Here's how the part is built. I have some questions about the finished solid (model axes, mm). A direction names the side the tool comes from. Round coordinates to 2 decimals unless told otherwise and drop trailing zeros. Order: outer loops, then holes, each group sorted by start corner. A loop starts at its lowest first (then second) coordinate and runs counter-clockwise, first axis right, second up. Notation, with made-up numbers: (-18.5, 72) -> (15.5, 72) arc R31 cw to (15.5, 103) -> close; hole circle Ø9 at (37, -3). An arc over 180 degrees is marked (long way). Use a Markdown table: item, result. Add a question column.
(1) I want a section at B-B, the plane z = 91. Please give me the cut outline in (x, y).
(2) If I drill on probe 1 along Z at (x, y) = (-15, -3.7); probe 2 along Z at (x, y) = (15, -5); probe 3 along Z at (x, y) = (12, -0.25), over which ranges is the centre line in solid material (lowest first)?
(3) On a 3-axis mill with a long thin cutter (end or side, diameter ignored), from which of +Z, -Z, +X, -X, +Y, -Y can I reach the whole of each face in a straight line? I mean faces 4 (the face through (21, -12, 48)), 5 (the face through (9.5, -5, 6)), 6 (the face through (-4, -6, 75.5)), 7 (the face through (0, -6.2, 47.5)), 8 (the face through (-13.9, -3, 33.9)). Say none if no direction works.
(4) I'm going to push flat-ended pins straight in: P1, Ø2, axis at y = -8.5, z = 70.5, coming from the -X side; P2, Ø6, axis at x = 12.5, z = 20, coming from the -Y side; P3, Ø3.5, axis at x = -4, y = -9, coming from the +Z side. Where does each tip first touch, or does it pass through?
(5) I want a section at C-C, the plane x = 0. Please give me the cut outline in (y, z), then the cut area to 3 significant figures.
(6) Thinking about a two-plate mould opening in X: for faces 1 (the face through (-21.843, -2, 48)), 2 (the face through (-13.6, -1.48, 62.06)), 3 (the face through (-17, -4, 48)), which applies, pulls with the +X half, pulls with the -X half, needs draft (parallel to the pull), parting line crosses it, or undercut?
(7) I want a section at D-D, the plane z = 62. Please give me the cut outline in (x, y).
(8) I want a section at A-A, the plane x = 15. Please give me the cut outline in (y, z).
from build123d import *

# Parameters (mm, degrees)
SKETCH012_R  = 4
PAD008_DEPTH = 12
SKETCH001_R  = 1.4
SKETCH001_W  = 29.46
SKETCH001_H  = 21.5
PAD005_DEPTH = 13
PAD006_DEPTH = 24
SKETCH010_R  = 2.5
PAD007_DEPTH = 4
SKETCH011_R  = 2.5
PAD004_DEPTH = 1
PAD001_DEPTH = 1
PAD002_DEPTH = 2
PAD003_DEPTH = 1
PAD_DEPTH    = 97


with BuildPart() as pad008:
    # Sketch012 → Pad008 (new body)
    with BuildSketch(Plane.XZ):
        with Locations((30, 65)):
            Circle(SKETCH012_R)
    extrude(amount=PAD008_DEPTH)


with BuildPart() as pad005:
    # Sketch001 → Pad005 (new body)
    with BuildSketch(Plane(origin=(0, 0, 0), x_dir=(-1, 0, 0), z_dir=(0, 1, 0))):
        with Locations((15, 62)):
            Circle(SKETCH001_R)
        with Locations((15, 35)):
            Circle(SKETCH001_R)
        with Locations((-15, 62)):
            Circle(SKETCH001_R)
        with Locations((-15, 35)):
            Circle(SKETCH001_R)
        with Locations((7.27, 10.75)):
            Rectangle(SKETCH001_W, SKETCH001_H)
        with Locations((7.27, 86.25)):
            Rectangle(SKETCH001_W, SKETCH001_H)
    extrude(amount=-PAD005_DEPTH)


with BuildPart() as pad006:
    # Sketch008 → Pad006 (new body)
    with BuildSketch(Plane.YZ.offset(33.5)):
        with BuildLine():
            ThreePointArc((-1, 7.5), (-8.915757, 6), (-1, 4.5))
            Line((0, 4.5), (-1, 4.5))
            Line((0, 7.5), (0, 4.5))
            Line((-1, 7.5), (0, 7.5))
        make_face()
        with BuildLine():
            ThreePointArc((-1, 92.5), (-8.915757, 91), (-1, 89.5))
            Line((0, 89.5), (-1, 89.5))
            Line((0, 92.5), (0, 89.5))
            Line((-1, 92.5), (0, 92.5))
        make_face()
    extrude(amount=-PAD006_DEPTH)


with BuildPart() as pad007:
    # Sketch010 → Pad007 (new body)
    with BuildSketch(Plane.XZ.offset(12)):
        with Locations((15, 62)):
            Circle(SKETCH010_R)
        with Locations((15, 35)):
            Circle(SKETCH010_R)
    extrude(amount=-PAD007_DEPTH)


with BuildPart() as cutblock:
    # Sketch011 → Pad004 (new body)
    with BuildSketch(Plane.XZ.offset(4)):
        with Locations((-15, 62)):
            Circle(SKETCH011_R)
        with Locations((-15, 35)):
            Circle(SKETCH011_R)
    extrude(amount=-PAD004_DEPTH)

    # Fusion001: union Pad005, Pad006, Pad007
    add(pad005.part)
    add(pad006.part)
    add(pad007.part)


with BuildPart() as pad001:
    # Sketch005 → Pad001 (new body)
    with BuildSketch(Plane(origin=(0, 0, 21.5), x_dir=(-1, 0, 0), z_dir=(0, 0, 1))):
        with BuildLine():
            ThreePointArc((7.46, 0), (0, 7.46), (-7.46, 0))
            Line((-7.46, 0), (-6, 0))
            ThreePointArc((6, 0), (0, 6), (-6, 0))
            Line((7.46, 0), (6, 0))
        make_face()
    extrude(amount=PAD001_DEPTH)


with BuildPart() as pad002:
    # Sketch006 → Pad002 (new body)
    with BuildSketch(Plane(origin=(0, 0, 47.5), x_dir=(-1, 0, 0), z_dir=(0, 0, 1))):
        with BuildLine():
            ThreePointArc((7.46, 0), (0, 7.46), (-7.46, 0))
            Line((-7.46, 0), (-6, 0))
            ThreePointArc((6, 0), (0, 6), (-6, 0))
            Line((7.46, 0), (6, 0))
        make_face()
    extrude(amount=PAD002_DEPTH)


with BuildPart() as pad003:
    # Sketch007 → Pad003 (new body)
    with BuildSketch(Plane(origin=(0, 0, 74.5), x_dir=(-1, 0, 0), z_dir=(0, 0, 1))):
        with BuildLine():
            ThreePointArc((7.46, 0), (0, 7.46), (-7.46, 0))
            Line((-7.46, 0), (-6, 0))
            ThreePointArc((6, 0), (0, 6), (-6, 0))
            Line((7.46, 0), (6, 0))
        make_face()
    extrude(amount=PAD003_DEPTH)


with BuildPart() as cut001:
    # Sketch → Pad (new body)
    with BuildSketch(Plane.XY):
        with BuildLine():
            ThreePointArc((-7.46, 0), (0, -7.46), (7.46, 0))
            Line((7.46, 0), (40, 0))
            Line((40, -12), (40, 0))
            Line((3.5, -12), (40, -12))
            ThreePointArc((-11.842719, -4), (-5.779294, -11.083761), (3.5, -12))
            Line((-21.842719, -4), (-11.842719, -4))
            Line((-21.842719, 0), (-21.842719, -4))
            Line((-7.46, 0), (-21.842719, 0))
        make_face()
    extrude(amount=PAD_DEPTH)

    # Fusion: union Pad001, Pad002, Pad003
    add(pad001.part)
    add(pad002.part)
    add(pad003.part)

    # Cut: cut CutBlock
    add(cutblock.part, mode=Mode.SUBTRACT)

    # Cut001: cut Pad008
    add(pad008.part, mode=Mode.SUBTRACT)


solid = cut001.part
Taken from the geometry:
| question | item | result |
|---|---|---|
| 1 | outline | (7.46, -12) -> (40, -12) -> (40, 0) -> (33.5, 0) -> (33.5, -8.92) -> (9.5, -8.92) -> (9.5, 0) -> (7.46, 0) -> close |
| 2 | probe 1 | z = 21.5 to 32.5, 37.5 to 59.5, 64.5 to 75.5 |
| 2 | probe 2 | z = 0 to 1.9, 10.1 to 33.6, 36.4 to 60.6, 63.4 to 86.9, 95.1 to 97 |
| 2 | probe 3 | z = 0 to 4.5, 7.5 to 89.5, 92.5 to 97 |
| 3 | face 4 | +Z, -Z, +X, -Y |
| 3 | face 5 | none |
| 3 | face 6 | +Z, -X, +Y, -Y |
| 3 | face 7 | +Y |
| 3 | face 8 | -Y |
| 4 | P1 | stops at x = -10 |
| 4 | P2 | stops at y = -12 |
| 4 | P3 | stops at z = 75.5 |
| 5 | outline | (-12.5, 21.5) -> (-6, 21.5) -> (-6, 22.5) -> (-7.46, 22.5) -> (-7.46, 47.5) -> (-6, 47.5) -> (-6, 49.5) -> (-7.46, 49.5) -> (-7.46, 74.5) -> (-6, 74.5) -> (-6, 75.5) -> (-12.5, 75.5) -> close |
| 5 | area | 278 mm2 |
| 6 | face 1 | pulls with the -X half |
| 6 | face 2 | undercut |
| 6 | face 3 | needs draft |
| 7 | outline | (-21.84, -4) -> (-17.5, -4) -> (-17.5, -3) -> (-16.4, -3) -> (-16.4, 0) -> (-21.84, 0) -> close; (-13.6, -3) -> (-12.5, -3) -> (-12.5, -4) -> (-11.84, -4) arc R12.5 ccw to (3.5, -12) -> (12.5, -12) -> (12.5, -8) -> (13.6, -8) -> (13.6, 0) -> (7.46, 0) arc R7.46 cw to (-7.46, 0) -> (-13.6, 0) -> close; (16.4, -8) -> (17.5, -8) -> (17.5, -12) -> (27.35, -12) -> (27.35, 0) -> (16.4, 0) -> close; (32.65, -12) -> (40, -12) -> (40, 0) -> (32.65, 0) -> close |
| 8 | outline | (-12, 0) -> (0, 0) -> (0, 4.5) -> (-1, 4.5) arc R4.1 cw (long way) to (-1, 7.5) -> (0, 7.5) -> (0, 33.6) -> (-8, 33.6) -> (-8, 32.5) -> (-12, 32.5) -> close; (-12, 37.5) -> (-8, 37.5) -> (-8, 36.4) -> (0, 36.4) -> (0, 60.6) -> (-8, 60.6) -> (-8, 59.5) -> (-12, 59.5) -> close; (-12, 64.5) -> (-8, 64.5) -> (-8, 63.4) -> (0, 63.4) -> (0, 89.5) -> (-1, 89.5) arc R4.1 cw (long way) to (-1, 92.5) -> (0, 92.5) -> (0, 97) -> (-12, 97) -> close |
